Geometry check sheet. Reference: the model listing, model coordinates, mm. Coordinates: 2 decimals unless noted, no trailing zeros. Write each loop counter-clockwise with the first axis right and the second up, starting at its lowest first coordinate (ties: lowest second). Pieces come first, ordered by that corner, then holes. Notation, with made-up numbers: M 34,69 L 65,69 A25 ccw 65,100 Z; hole C -21,5.25 d7. An arc over 180 degrees is marked long. Answer as a JSON object with one key per item and string values. Group by question number.
```python
from build123d import *

# Parameters (mm, degrees)
SKETCH1_W           = 40
SKETCH1_H           = 60
BOSS_EXTRUDE1_DEPTH = 3.05
SKETCH4_W           = 3.3
SKETCH4_H           = 52
SKETCH4_W_2         = 3
SKETCH4_H_2         = 0.8
CUT_EXTRUDE1_DEPTH  = 10
CUT_EXTRUDE3_DEPTH  = 10
SKETCH7_R           = 1.5
CUT_EXTRUDE4_DEPTH  = 10


with BuildPart() as part:
    # Sketch1 → Boss-Extrude1 (new body)
    with BuildSketch(Plane(origin=(0, 0, 0), x_dir=(1, 0, 0), z_dir=(0, 1, 0))):
        with Locations((20, 30)):
            Rectangle(SKETCH1_W, SKETCH1_H)
    extrude(amount=BOSS_EXTRUDE1_DEPTH)

    # Sketch4 → Cut-Extrude1 (cut)
    with BuildSketch(Plane(origin=(0, 3.05, 0), x_dir=(1, 0, 0), z_dir=(0, 1, 0))):
        with Locations((20, 30)):
            Rectangle(SKETCH4_W, SKETCH4_H)
        with Locations((20, 57.6)):
            Rectangle(SKETCH4_W_2, SKETCH4_H_2)
    extrude(amount=-CUT_EXTRUDE1_DEPTH, mode=Mode.SUBTRACT)

    # Sketch6 → Cut-Extrude3 (cut)
    with BuildSketch(Plane(origin=(0, 3.05, 0), x_dir=(1, 0, 0), z_dir=(0, 1, 0))):
        Polygon((0, 60), (0, 35), (16.5, 35), (16.5, 39), (15, 39), (15, 43), (16.5, 43), (16.5, 60), align=None)
        Polygon((40, 60), (40, 35), (23.5, 35), (23.5, 39), (25, 39), (25, 43), (23.5, 43), (23.5, 60), align=None)
    extrude(amount=-CUT_EXTRUDE3_DEPTH, mode=Mode.SUBTRACT)

    # Sketch7 → Cut-Extrude4 (cut)
    with BuildSketch(Plane(origin=(0, 3.05, 0), x_dir=(1, 0, 0), z_dir=(0, 1, 0))):
        with Locations(Location((8, 2.5, 0), (0, 0, 270))):
            Circle(SKETCH7_R)
        with Locations(Location((32, 2.5, 0), (0, 0, 270))):
            Circle(SKETCH7_R)
    extrude(amount=-CUT_EXTRUDE4_DEPTH, mode=Mode.SUBTRACT)


solid = part.part
```
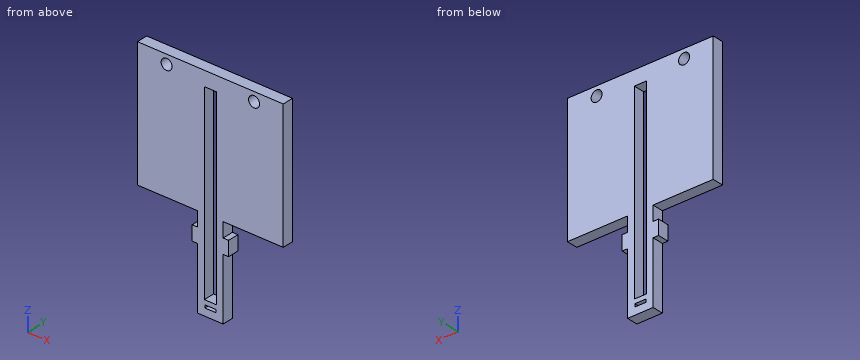
1) Material ranges on probe 1 along X at (y, z) = (1.25, -2.5); probe 2 along X at (y, z) = (0.65, -52); probe 3 along X at (y, z) = (1.8, -3.5), recorded low to high. Write a range as [from, to].
2) Section check C-C (z = -10). Record the cut outline in (x, y), then the cut area to 3 significant figures.
3) Section check D-D (x = 32). Record the cut outline in (y, z).
4) Section check A-A (z = -2.5). Record the cut outline in (x, y), then the cut area to 3 significant figures.
5) Go/stop test with flat-tipped pins: pin 1 Ø1.5 at (y, z) = (1.5, -40.5) entering from -X; pin 2 Ø0.9 at (x, y) = (31, 1) entering from -Z; pin 3 Ø0.6 at (y, z) = (2, -57.5) entering from -X. Record where each tip stops, or that it passes through.
6) Section check B-B (y = 1.5). Record the cut outline in (x, z).
Entries:
{
 "1": {"probe 1": "[0, 6.5], [9.5, 30.5], [33.5, 40]", "probe 2": "[16.5, 18.35], [21.65, 23.5]", "probe 3": "[0, 6.88], [9.12, 30.88], [33.12, 40]"},
 "2": {"outline": "M 0,0 L 18.35,0 L 18.35,3.05 L 0,3.05 Z; M 21.65,0 L 40,0 L 40,3.05 L 21.65,3.05 Z", "area": "112 mm^2"},
 "3": {"outline": "M 0,-35 L 3.05,-35 L 3.05,-4 L 0,-4 Z; M 0,-1 L 3.05,-1 L 3.05,0 L 0,0 Z"},
 "4": {"outline": "M 0,0 L 6.5,0 L 6.5,3.05 L 0,3.05 Z; M 9.5,0 L 30.5,0 L 30.5,3.05 L 9.5,3.05 Z; M 33.5,0 L 40,0 L 40,3.05 L 33.5,3.05 Z", "area": "104 mm^2"},
 "5": {"pin 1": "x = 15", "pin 2": "z = -35", "pin 3": "x = 16.5"},
 "6": {"outline": "M 0,-35 L 16.5,-35 L 16.5,-39 L 15,-39 L 15,-43 L 16.5,-43 L 16.5,-60 L 23.5,-60 L 23.5,-43 L 25,-43 L 25,-39 L 23.5,-39 L 23.5,-35 L 40,-35 L 40,0 L 0,0 Z; hole C 8,-2.5 d3; hole M 18.35,-56 L 21.65,-56 L 21.65,-4 L 18.35,-4 Z; hole M 18.5,-58 L 21.5,-58 L 21.5,-57.2 L 18.5,-57.2 Z; hole C 32,-2.5 d3"}
}
